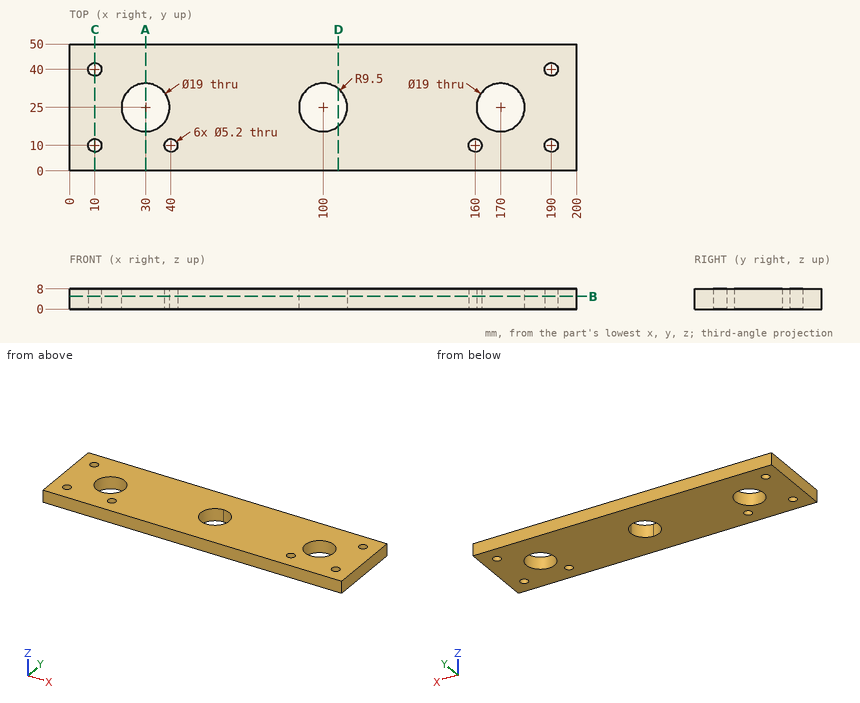
Could you check a few things on this drawing? It's one solid part, dimensions in mm from its lowest x, y, z. Coordinates: 2 decimals unless noted, no trailing zeros. Loops run counter-clockwise (first coordinate to the right, second up) from the corner with the lowest first, then second, coordinate; pieces in that order, holes last.
1. Imagine slicing it at D-D (x = 106). Please give me the cut outline in (y, z), and give its area (3 significant figures).
2. I need wall thicknesses on L1, parallel to Y at x = 10, z = 4.75; L2, parallel to Y at x = 40, z = 5.25; L3, parallel to X at y = 39, z = 5.5. Which ranges of each line are inside material? Lowest first, please.
3. Imagine slicing it at A-A (x = 30). Please give me the cut outline in (y, z).
4. Imagine slicing it at C-C (x = 10). Please give me the cut outline in (y, z), and give its area (3 significant figures).
5. Imagine slicing it at B-B (z = 5). Give the number of separate pieces and of enclosed holes in the cut face, and give its area (3 significant figures).
Computed values:
1. outline: (0, 0) - (17.63, 0) - (17.63, 8) - (0, 8) - close; (32.37, 0) - (50, 0) - (50, 8) - (32.37, 8) - close
1. area: 282 mm2
2. L1: y = 0 to 7.4, 12.6 to 37.4, 42.6 to 50
2. L2: y = 0 to 7.4, 12.6 to 50
2. L3: x = 0 to 7.6, 12.4 to 187.6, 192.4 to 200
3. outline: (0, 0) - (15.5, 0) - (15.5, 8) - (0, 8) - close; (34.5, 0) - (50, 0) - (50, 8) - (34.5, 8) - close
4. outline: (0, 0) - (7.4, 0) - (7.4, 8) - (0, 8) - close; (12.6, 0) - (37.4, 0) - (37.4, 8) - (12.6, 8) - close; (42.6, 0) - (50, 0) - (50, 8) - (42.6, 8) - close
4. area: 317 mm2
5. separate pieces: 1
5. enclosed holes: 9
5. area: 9,020 mm2
